CAD build for the part. Positions are in the model's coordinates, mm. Coordinates: 2 decimals unless noted, no trailing zeros. Order: outer loops, then holes, each group sorted by start corner. A loop starts at its lowest first (then second) coordinate and runs counter-clockwise, first axis right, second up. Notation, with made-up numbers: (24, -26) - (75, -26) arc R23 ccw to (75, 0) - close; hole circle Ø1 at (89, 29.25). An arc over 180 degrees is marked (long way). Use one line per item in the form item = value.
```python
from build123d import *

# Parameters (mm, degrees)
SKETCH1_R           = 2.2225
BOSS_EXTRUDE1_DEPTH = 3.175
SKETCH2_R           = 2.159
CUT_EXTRUDE1_DEPTH  = 297.247830215
CUT_EXTRUDE2_DEPTH  = 297.247830215
SKETCH7_R           = 1.524
CUT_EXTRUDE3_DEPTH  = 297.247830215
SKETCH10_R          = 2.159
CUT_EXTRUDE6_DEPTH  = 297.247830215
SKETCH9_R           = 2.032
CUT_EXTRUDE5_DEPTH  = 297.247830215
SKETCH13_R          = 1.1
CUT_EXTRUDE8_DEPTH  = 297.247830215
SKETCH14_R          = 3.175
CUT_EXTRUDE9_DEPTH  = 297.247830215
SKETCH15_R          = 2.159
CUT_EXTRUDE10_DEPTH = 297.247830215
SKETCH16_R          = 2.159
CUT_EXTRUDE11_DEPTH = 297.247830215


with BuildPart() as part:
    # Sketch1 → Boss-Extrude1 (new body)
    with BuildSketch(Plane(origin=(0, 0, 0), x_dir=(1, 0, 0), z_dir=(0, 1, 0))):
        Polygon((-85.365028143, 123.058976948), (-121.286052627, 87.137952464), (-121.286052627, -196.619998567), (-85.365028143, -232.541023052), (147.592922888, -232.541023052), (183.513947373, -196.619998567), (183.513947373, 87.137952464), (147.592922888, 123.058976948), align=None)
        with Locations(Location((-16.765052627, -213.491023052, 0), (0, 0, 270))):
            Circle(SKETCH1_R, mode=Mode.SUBTRACT)
        with Locations(Location((-16.765052627, -171.581023052, 0), (0, 0, 270))):
            Circle(SKETCH1_R, mode=Mode.SUBTRACT)
        with Locations(Location((-16.765052627, -75.696023052, 0), (0, 0, 270))):
            Circle(SKETCH1_R, mode=Mode.SUBTRACT)
        with Locations(Location((78.992947373, -213.491023052, 0), (0, 0, 270))):
            Circle(SKETCH1_R, mode=Mode.SUBTRACT)
        with Locations(Location((78.992947373, -171.581023052, 0), (0, 0, 270))):
            Circle(SKETCH1_R, mode=Mode.SUBTRACT)
        with Locations(Location((78.992947373, -75.696023052, 0), (0, 0, 270))):
            Circle(SKETCH1_R, mode=Mode.SUBTRACT)
        with Locations(Location((-16.765052627, -33.786023052, 0), (0, 0, 270))):
            Circle(SKETCH1_R, mode=Mode.SUBTRACT)
        with Locations(Location((-16.765052627, 62.098976948, 0), (0, 0, 270))):
            Circle(SKETCH1_R, mode=Mode.SUBTRACT)
        with Locations(Location((-16.765052627, 104.008976948, 0), (0, 0, 270))):
            Circle(SKETCH1_R, mode=Mode.SUBTRACT)
        with Locations(Location((78.992947373, -33.786023052, 0), (0, 0, 270))):
            Circle(SKETCH1_R, mode=Mode.SUBTRACT)
        with Locations(Location((78.992947373, 62.098976948, 0), (0, 0, 270))):
            Circle(SKETCH1_R, mode=Mode.SUBTRACT)
        with Locations(Location((78.992947373, 104.008976948, 0), (0, 0, 270))):
            Circle(SKETCH1_R, mode=Mode.SUBTRACT)
    extrude(amount=BOSS_EXTRUDE1_DEPTH)

    # Sketch2 → Cut-Extrude1 (cut, through all)
    with BuildSketch(Plane(origin=(0, 3.175, 0), x_dir=(1, 0, 0), z_dir=(0, 1, 0))):
        with Locations(Location((13.841947373, -12.069023052, 0), (0, 0, 270))):
            Circle(SKETCH2_R)
        with Locations(Location((48.131947373, -12.069023052, 0), (0, 0, 270))):
            Circle(SKETCH2_R)
        with Locations(Location((13.841947373, -97.159023052, 0), (0, 0, 270))):
            Circle(SKETCH2_R)
        with Locations(Location((48.131947373, -97.159023052, 0), (0, 0, 270))):
            Circle(SKETCH2_R)
    extrude(amount=-CUT_EXTRUDE1_DEPTH, mode=Mode.SUBTRACT)

    # Sketch4 → Cut-Extrude2 (cut, through all)
    with BuildSketch(Plane(origin=(0, 3.175, 0), x_dir=(1, 0, 0), z_dir=(0, 1, 0))):
        with BuildLine():
            Line((-0.636052627, 51.430976948), (62.863947373, 51.430976948))
            ThreePointArc((62.863947373, 51.430976948), (66.038947373, 48.255976948), (62.863947373, 45.080976948))
            Line((62.863947373, 45.080976948), (-0.636052627, 45.080976948))
            ThreePointArc((-0.636052627, 45.080976948), (-3.811052627, 48.255976948), (-0.636052627, 51.430976948))
        make_face()
        with BuildLine():
            Line((-0.636052627, 0.630976948), (62.863947373, 0.630976948))
            ThreePointArc((62.863947373, 0.630976948), (66.038947373, -2.544023052), (62.863947373, -5.719023052))
            Line((62.863947373, -5.719023052), (-0.636052627, -5.719023052))
            ThreePointArc((-0.636052627, -5.719023052), (-3.811052627, -2.544023052), (-0.636052627, 0.630976948))
        make_face()
        with BuildLine():
            Line((-0.636052627, -110.113023052), (62.863947373, -110.113023052))
            ThreePointArc((62.863947373, -110.113023052), (66.038947373, -106.938023052), (62.863947373, -103.763023052))
            Line((62.863947373, -103.763023052), (-0.636052627, -103.763023052))
            ThreePointArc((-0.636052627, -103.763023052), (-3.811052627, -106.938023052), (-0.636052627, -110.113023052))
        make_face()
        with BuildLine():
            Line((-0.636052627, -160.913023052), (62.863947373, -160.913023052))
            ThreePointArc((62.863947373, -160.913023052), (66.038947373, -157.738023052), (62.863947373, -154.563023052))
            Line((62.863947373, -154.563023052), (-0.636052627, -154.563023052))
            ThreePointArc((-0.636052627, -154.563023052), (-3.811052627, -157.738023052), (-0.636052627, -160.913023052))
        make_face()
    extrude(amount=-CUT_EXTRUDE2_DEPTH, mode=Mode.SUBTRACT)

    # Sketch7 → Cut-Extrude3 (cut, through all)
    with BuildSketch(Plane(origin=(0, 3.175, 0), x_dir=(1, 0, 0), z_dir=(0, 1, 0))):
        with Locations(Location((16.127947373, 67.686976948, 0), (0, 0, 270))):
            Circle(SKETCH7_R)
        with Locations(Location((46.099947373, 67.686976948, 0), (0, 0, 270))):
            Circle(SKETCH7_R)
        with Locations(Location((16.127947373, 97.658976948, 0), (0, 0, 270))):
            Circle(SKETCH7_R)
        with Locations(Location((46.099947373, 97.658976948, 0), (0, 0, 270))):
            Circle(SKETCH7_R)
    extrude(amount=-CUT_EXTRUDE3_DEPTH, mode=Mode.SUBTRACT)

    # Sketch10 → Cut-Extrude6 (cut, through all)
    with BuildSketch(Plane.XZ):
        with Locations(Location((6.983947373, 193.475823052, 0), (0, 0, 270))):
            Circle(SKETCH10_R)
        with Locations(Location((55.243947373, 193.475823052, 0), (0, 0, 270))):
            Circle(SKETCH10_R)
        with Locations(Location((6.983947373, 169.345823052, 0), (0, 0, 270))):
            Circle(SKETCH10_R)
        with Locations(Location((55.243947373, 169.345823052, 0), (0, 0, 270))):
            Circle(SKETCH10_R)
    extrude(amount=-CUT_EXTRUDE6_DEPTH, mode=Mode.SUBTRACT)

    # Sketch9 → Cut-Extrude5 (cut, through all)
    with BuildSketch(Plane(origin=(0, 0, 0), x_dir=(-1, 0, 0), z_dir=(0, -1, 0))):
        with Locations(Location((-69.213947373, -200.791023052, 0), (0, 0, 90))):
            Circle(SKETCH9_R)
        with Locations(Location((-96.645947373, -200.791023052, 0), (0, 0, 90))):
            Circle(SKETCH9_R)
        with Locations(Location((-69.213947373, -171.835023052, 0), (0, 0, 90))):
            Circle(SKETCH9_R)
        with Locations(Location((-96.645947373, -171.835023052, 0), (0, 0, 90))):
            Circle(SKETCH9_R)
    extrude(amount=-CUT_EXTRUDE5_DEPTH, mode=Mode.SUBTRACT)

    # Sketch13 → Cut-Extrude8 (cut, through all)
    with BuildSketch(Plane.XZ):
        with Locations(Location((16.113947373, 69.741023052, 0), (0, 0, 270))):
            Circle(SKETCH13_R)
        with Locations(Location((16.113947373, 39.741023052, 0), (0, 0, 270))):
            Circle(SKETCH13_R)
        with Locations(Location((46.113947373, 39.741023052, 0), (0, 0, 90))):
            Circle(SKETCH13_R)
        with Locations(Location((46.113947373, 69.741023052, 0), (0, 0, 90))):
            Circle(SKETCH13_R)
    extrude(amount=-CUT_EXTRUDE8_DEPTH, mode=Mode.SUBTRACT)

    # Sketch14 → Cut-Extrude9 (cut, through all)
    with BuildSketch(Plane.XZ):
        with Locations(Location((-103.325540385, 196.619998567, 0), (0, 0, 270))):
            Circle(SKETCH14_R)
        with Locations(Location((-85.365028143, 214.580510809, 0), (0, 0, 270))):
            Circle(SKETCH14_R)
        with Locations(Location((-85.365028143, 178.659486325, 0), (0, 0, 270))):
            Circle(SKETCH14_R)
        with Locations(Location((-67.404515901, 196.619998567, 0), (0, 0, 270))):
            Circle(SKETCH14_R)
        with Locations(Location((129.632410646, 196.619998567, 0), (0, 0, 90))):
            Circle(SKETCH14_R)
        with Locations(Location((147.592922888, 178.659486325, 0), (0, 0, 90))):
            Circle(SKETCH14_R)
        with Locations(Location((165.55343513, 196.619998567, 0), (0, 0, 90))):
            Circle(SKETCH14_R)
        with Locations(Location((147.592922888, 214.580510809, 0), (0, 0, 90))):
            Circle(SKETCH14_R)
        with Locations(Location((-85.365028143, -105.098464706, 0), (0, 0, 90))):
            Circle(SKETCH14_R)
        with Locations(Location((-103.325540385, -87.137952464, 0), (0, 0, 90))):
            Circle(SKETCH14_R)
        with Locations(Location((-85.365028143, -69.177440222, 0), (0, 0, 90))):
            Circle(SKETCH14_R)
        with Locations(Location((-67.404515901, -87.137952464, 0), (0, 0, 90))):
            Circle(SKETCH14_R)
        with Locations(Location((165.55343513, -87.137952464, 0), (0, 0, 270))):
            Circle(SKETCH14_R)
        with Locations(Location((147.592922888, -69.177440222, 0), (0, 0, 270))):
            Circle(SKETCH14_R)
        with Locations(Location((147.592922888, -105.098464706, 0), (0, 0, 270))):
            Circle(SKETCH14_R)
        with Locations(Location((129.632410646, -87.137952464, 0), (0, 0, 270))):
            Circle(SKETCH14_R)
    extrude(amount=-CUT_EXTRUDE9_DEPTH, mode=Mode.SUBTRACT)

    # Sketch15 → Cut-Extrude10 (cut, through all)
    with BuildSketch(Plane.XZ):
        with Locations(Location((5.713947373, 222.381023052, 0), (0, 0, 270))):
            Circle(SKETCH15_R)
        with Locations(Location((-45.086052627, 222.381023052, 0), (0, 0, 270))):
            Circle(SKETCH15_R)
        with Locations(Location((-111.126052627, 54.741023052, 0), (0, 0, 270))):
            Circle(SKETCH15_R)
        with Locations(Location((-111.126052627, 105.541023052, 0), (0, 0, 270))):
            Circle(SKETCH15_R)
        with Locations(Location((-111.126052627, 156.341023052, 0), (0, 0, 270))):
            Circle(SKETCH15_R)
        with Locations(Location((173.353947373, 156.341023052, 0), (0, 0, 90))):
            Circle(SKETCH15_R)
        with Locations(Location((173.353947373, 105.541023052, 0), (0, 0, 90))):
            Circle(SKETCH15_R)
        with Locations(Location((173.353947373, 54.741023052, 0), (0, 0, 90))):
            Circle(SKETCH15_R)
        with Locations(Location((107.313947373, 222.381023052, 0), (0, 0, 90))):
            Circle(SKETCH15_R)
        with Locations(Location((56.513947373, 222.381023052, 0), (0, 0, 90))):
            Circle(SKETCH15_R)
        with Locations(Location((56.513947373, -112.898976948, 0), (0, 0, 270))):
            Circle(SKETCH15_R)
        with Locations(Location((107.313947373, -112.898976948, 0), (0, 0, 270))):
            Circle(SKETCH15_R)
        with Locations(Location((173.353947373, 3.941023052, 0), (0, 0, 270))):
            Circle(SKETCH15_R)
        with Locations(Location((173.353947373, -46.858976948, 0), (0, 0, 270))):
            Circle(SKETCH15_R)
        with Locations(Location((-111.126052627, -46.858976948, 0), (0, 0, 90))):
            Circle(SKETCH15_R)
        with Locations(Location((-111.126052627, 3.941023052, 0), (0, 0, 90))):
            Circle(SKETCH15_R)
        with Locations(Location((-45.086052627, -112.898976948, 0), (0, 0, 90))):
            Circle(SKETCH15_R)
        with Locations(Location((5.713947373, -112.898976948, 0), (0, 0, 90))):
            Circle(SKETCH15_R)
    extrude(amount=-CUT_EXTRUDE10_DEPTH, mode=Mode.SUBTRACT)

    # Sketch16 → Cut-Extrude11 (cut, through all)
    with BuildSketch(Plane(origin=(0, 0, 0), x_dir=(-1, 0, 0), z_dir=(0, -1, 0))):
        with Locations(Location((-133.333707373, -106.679409794, 0), (0, 0, 90))):
            Circle(SKETCH16_R)
        with Locations(Location((-138.413707373, -4.529409794, 0), (0, 0, 90))):
            Circle(SKETCH16_R)
        with Locations(Location((-160.653947373, -53.029409794, 0), (0, 0, 90))):
            Circle(SKETCH16_R)
    extrude(amount=-CUT_EXTRUDE11_DEPTH, mode=Mode.SUBTRACT)


solid = part.part
```
Item 1: Drill centre lines: line 1 (X direction, y = 2.3, z = 76); line 2 (Z direction, x = -44, y = 2.4); line 3 (Z direction, x = -85.5, y = 2.1). Where is each one in solid material? Low to high. Write a range as [from, to].
Derived:
line_1 = [-121.29, -18.97], [-14.56, 76.79], [81.19, 183.51]
line_2 = [-123.06, -114.76], [-111.03, 220.52], [224.25, 232.54]
line_3 = [-122.92, -108.27], [-101.93, -72.35], [-66.01, 175.49], [181.83, 211.41], [217.75, 232.41]
Item 2: Cut at A-A, the plane x = 40. Write the cut outline in (y, z) (3 decimals), plus the area to 3 significant figures.
Derived:
outline = (0, -123.059) - (3.175, -123.059) - (3.175, -51.431) - (0, -51.431) - close; (0, -45.081) - (3.175, -45.081) - (3.175, -0.631) - (0, -0.631) - close; (0, 5.719) - (3.175, 5.719) - (3.175, 103.763) - (0, 103.763) - close; (0, 110.113) - (3.175, 110.113) - (3.175, 154.563) - (0, 154.563) - close; (0, 160.913) - (3.175, 160.913) - (3.175, 232.541) - (0, 232.541) - close
area = 1,050 mm²
Item 3: Cut at B-B, the plane y = 2.6. State how many separate pieces and enclosed holes the cut face has, plus the area to 3 significant figures.
Derived:
separate_pieces = 1
enclosed_holes = 73
area = 103,000 mm²
Item 4: Drop a flat-ended pin along its axis: pin 1 (3.5 mm diameter, centred on x = 69.21, z = 171.84, fed in from +Y). Give the stop position or say it passes through.
Derived:
pin_1 = through
